Geometry check sheet. Reference: drawing and pictorial views, mm from the part's lowest x, y, z. Round coordinates to 2 decimals unless told otherwise and drop trailing zeros. Order: outer loops, then holes, each group sorted by start corner. A loop starts at its lowest first (then second) coordinate and runs counter-clockwise, first axis right, second up. Notation, with made-up numbers: (-7, 69) -> (39, 69) arc R18 ccw to (39, 75) -> close; hole circle Ø1 at (71.25, -24.75). An arc over 180 degrees is marked (long way). Put each result on its own line as item: value.
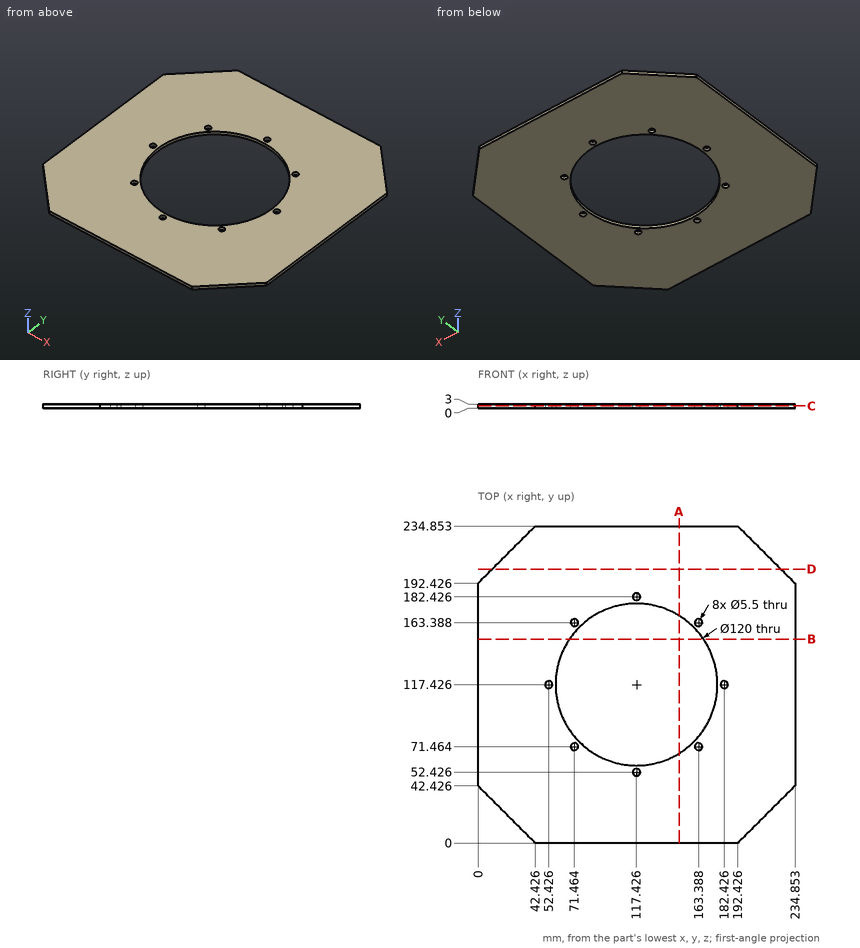
Item 1: Sectioned sample at C-C, the plane z = 1.6. Give the number of separate pieces and of enclosed holes in the cut face, then the cut area to 3 significant figures.
Geometry check:
separate pieces: 1
enclosed holes: 9
area: 40,100 mm2
Item 2: Sectioned sample at B-B, the plane y = 151. Record the boundary of the cut face in (x, z).
Geometry check:
outline: (0, 0) -> (67.7, 0) -> (67.7, 3) -> (0, 3) -> close; (167.15, 0) -> (234.85, 0) -> (234.85, 3) -> (167.15, 3) -> close
Item 3: Sectioned sample at D-D, the plane y = 203. Record the boundary of the cut face in (x, z).
Geometry check:
outline: (10.57, 0) -> (224.28, 0) -> (224.28, 3) -> (10.57, 3) -> close
Item 4: Material ranges on line 1 along Y through (x, z) = (101, 2.05) (1 decimal); line 2 along Y through (x, z) = (122, 2.75); line 3 along X through (y, z) = (112, 0.15), recorded low to high.
Geometry check:
line 1: 0 to 59.7, 175.1 to 234.9
line 2: 0 to 57.6, 177.25 to 234.85
line 3: 0 to 57.67, 177.18 to 234.85
Item 5: Sectioned sample at A-A, the plane x = 149. Record the boundary of the cut face in (y, z) (1 decimal).
Geometry check:
outline: (0, 0) -> (66.4, 0) -> (66.4, 3) -> (0, 3) -> close; (168.4, 0) -> (234.9, 0) -> (234.9, 3) -> (168.4, 3) -> close
Item 6: Depth check by flat-ended pin: pin 1 Ø4.5 at (x, y) = (182.43, 117.43) entering from -Z. Enter the tip coordinate at first touch or a pass-through.
Geometry check:
pin 1: through
